Design review of the part built by this model. Coordinates are the model's own, in mm. Face numbers are marked on the shaded views. A direction names the side the tool comes from. Give positions to 0.01 mm unless a question says otherwise; leave off trailing zeros. Write each loop counter-clockwise with the first axis right and the second up, starting at its lowest first coordinate (ties: lowest second). Pieces come first, ordered by that corner, then holes. Notation, with made-up numbers: (13.25, 85) -> (46.25, 85) arc R23 ccw to (46.25, 107) -> close; hole circle Ø10 at (-38, 36). An arc over 180 degrees is marked (long way). Use CSV: the item, a comma, the result in double quotes.
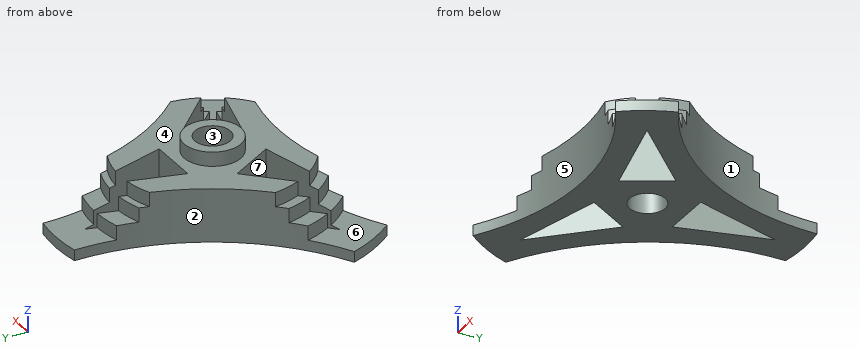
```python
from build123d import *

# Parameters (mm, degrees)
SKETCH_R              = 45
PAD_DEPTH             = 3
SKETCH001_R           = 33
PAD001_DEPTH          = 4
SKETCH002_R           = 28.25
PAD002_DEPTH          = 4
SKETCH003_R           = 25.9
PAD003_DEPTH          = 4
SKETCH004_R           = 8
PAD004_DEPTH          = 4
SKETCH005_R           = 5
POCKET_DEPTH          = 19.001
SKETCH006_R           = 66
POCKET001_DEPTH       = 276.380098
POLARPATTERN_COUNT    = 3
POCKET002_DEPTH       = 246.643698
POLARPATTERN001_COUNT = 3


with BuildPart() as part:
    # Sketch → Pad (new body)
    with BuildSketch(Plane.XY):
        with Locations((0.22389, -1.005935)):
            Circle(SKETCH_R)
    extrude(amount=PAD_DEPTH)

    # Sketch001 (on Face3 of Pad) → Pad001 (join)
    with BuildSketch(Plane.XY.offset(3)):
        Circle(SKETCH001_R)
    extrude(amount=PAD001_DEPTH)

    # Sketch002 (on Face5 of Pad001) → Pad002 (join)
    with BuildSketch(Plane.XY.offset(7)):
        with Locations((-0.334541, -0.419601)):
            Circle(SKETCH002_R)
    extrude(amount=PAD002_DEPTH)

    # Sketch003 (on Face7 of Pad002) → Pad003 (join)
    with BuildSketch(Plane.XY.offset(11)):
        Circle(SKETCH003_R)
    extrude(amount=PAD003_DEPTH)

    # Sketch004 (on Face9 of Pad003) → Pad004 (join)
    with BuildSketch(Plane.XY.offset(15)):
        Circle(SKETCH004_R)
    extrude(amount=PAD004_DEPTH)

    # Sketch005 (on Face2 of Pad004) → Pocket (cut, through all)
    with BuildSketch(Plane(origin=(0, 0, 0), x_dir=(1, 0, 0), z_dir=(0, 0, -1))):
        Circle(SKETCH005_R)
    extrude(amount=-POCKET_DEPTH, mode=Mode.SUBTRACT)

    # Sketch006 (on Face2 of Pocket) → Pocket001 (cut, through all)
    with BuildSketch(Plane(origin=(0, 0, 0), x_dir=(1, 0, 0), z_dir=(0, 0, -1))):
        with Locations((0, 85)):
            Circle(SKETCH006_R)
    pocket001 = extrude(amount=-POCKET001_DEPTH, mode=Mode.SUBTRACT)

    # PolarPattern: Pocket001 ×3 about axis
    polarpattern_axis = Axis((0, 0, 0), (0, 0, -1))
    for i in range(1, POLARPATTERN_COUNT):
        add(pocket001.rotate(polarpattern_axis, i * 360 / POLARPATTERN_COUNT), mode=Mode.SUBTRACT)

    # Sketch007 (on Face2 of PolarPattern) → Pocket002 (cut, through all)
    with BuildSketch(Plane(origin=(0, 0, 0), x_dir=(1, 0, 0), z_dir=(0, 0, -1))):
        Polygon((-7, -11), (7, -11), (0, -36), align=None)
    pocket002 = extrude(amount=-POCKET002_DEPTH, mode=Mode.SUBTRACT)

    # PolarPattern001: Pocket002 ×3 about axis
    polarpattern001_axis = Axis((0, 0, 0), (0, 0, -1))
    for i in range(1, POLARPATTERN001_COUNT):
        add(pocket002.rotate(polarpattern001_axis, i * 360 / POLARPATTERN001_COUNT), mode=Mode.SUBTRACT)


solid = part.part
```
(1) Take a section at B-B (y = 21). Write out the cut boundary in (x, z).
Established:
outline,"(-11.21, 0) -> (-4.2, 0) -> (-4.2, 15) -> (-11.21, 15) -> close; (4.2, 0) -> (11.21, 0) -> (11.21, 15) -> (4.2, 15) -> close"
(2) Mouldability with a two-part tool opening along X and no side actions: class the marked faces 1, 2 and 3 as +X half, -X half, draft (parallel to the pull), parting line (faces both ways), or undercut.
Established:
face 1,"+X half"
face 2,"-X half"
face 3,"undercut"
(3) Take a section at C-C (y = 13). Write out the cut boundary in (x, z), then the cut area to 3 significant figures.
Established:
outline,"(-14.57, 0) -> (-6.44, 0) -> (-6.44, 15) -> (-14.57, 15) -> close; (6.44, 0) -> (14.57, 0) -> (14.57, 15) -> (6.44, 15) -> close"
area,"244 mm2"
(4) Take a section at A-A (z = 13.5). Write out the cut boundary in (x, y), then the cut area to 3 significant figures.
Established:
outline,"(-25.73, -2.93) arc R25.9 ccw to (-23.73, -10.38) -> (-13.03, 0.56) -> (-6.03, -11.56) -> (-20.86, -15.36) arc R25.9 ccw to (-15.4, -20.82) arc R66 cw to (15.4, -20.82) arc R25.9 ccw to (20.86, -15.36) -> (6.03, -11.56) -> (13.03, 0.56) -> (23.73, -10.38) arc R25.9 ccw to (25.73, -2.93) arc R66 cw to (10.33, 23.75) arc R25.9 ccw to (2.87, 25.74) -> (7, 11) -> (-7, 11) -> (-2.87, 25.74) arc R25.9 ccw to (-10.33, 23.75) arc R66 cw to start; hole circle Ø10 at (0, 0)"
area,"1,160 mm2"
(5) Clearance check with flat-ended pins moving along their axes: pin 1 (3 mm diameter, centred on x = 4.5, y = 26, fed in from +Z); pin 2 (5 mm diameter, centred on x = 11, z = 12.5, fed in from -Y); pin 3 (9.5 mm diameter, centred on x = -3, y = 35, fed in from +Z). State where each tip first meets the part, or that it passes through.
Established:
pin 1,"stops at z = 15"
pin 2,"stops at y = -20.4"
pin 3,"stops at z = 7"
(6) Tool access review of the marked faces 4, 5, 6 and 7: name each direction out of +Z, -Z, +X, -X, +Y, -Y from which nothing blocks a thin tool from reaching the whole face with its end or side.
Established:
face 4,"+Z"
face 5,"+Z, -Z, -Y"
face 6,"+Z, -X, -Y"
face 7,"+Z, -Z"
(7) For line 1 along Y through (x, z) = (0, 11.5); line 2 along X through (y, z) = (0, 9.5); line 3 along Z through (x, y) = (-19.5, -17.5), list the stretches that pass through material, from the lowest coordinate up. Write a range as [from, to].
Established:
line 1,"y = [-19, -5], [5, 11]"
line 2,"x = [-23.12, -13.58], [-12.7, -5], [5, 12.7], [13.58, 23.12]"
line 3,"z = [0, 11]"
